Check sheet for the drawn part. Datum: minimum x, y, z corner. Units: mm. A direction names the side the tool comes from. Coordinates: 2 decimals unless noted, no trailing zeros. Order: outer loops, then holes, each group sorted by start corner. A loop starts at its lowest first (then second) coordinate and runs counter-clockwise, first axis right, second up. Notation, with made-up numbers: M 45.5,-7 L 96.5,-7 A18 ccw 96.5,25 Z; hole C 68,-12.5 d3. An arc over 180 degrees is marked long. Return JSON: item names as keys, results as strings. Group by question number.
Q1. Section check C-C, the plane x = 17. Enter the section's corners in (y, z).
Q2. Section check D-D, the plane y = 1. Enter the section's corners in (x, z), then the cut area to 3 significant figures.
Q3. Access from +Z, -Z, +X, -X, +Y, -Y to the whole of each face (thin tool, end or side, straight path). Record for the marked faces 1 and 2.
Q4. Go/stop test with flat-tipped pins: pin 1 Ø6 at (x, y) = (17.5, 7.5) entering from -Z; pin 2 Ø2 at (x, y) = (17, 5) entering from +Z; pin 3 Ø6 at (x, z) = (15.5, 6.5) entering from +Y. Record where each tip stops, or that it passes through.
Q5. Thickness scan on probe 1 along X at (y, z) = (13, 14.7); probe 2 along Y at (x, z) = (7, 14.6); probe 3 along X at (y, z) = (1.15, 7). Record the ranges inside material, lowest first.
Q6. Section check A-A, the plane y = 13. Enter the section's corners in (x, z).
Q7. Section check B-B, the plane z = 7. Enter the section's corners in (x, y).
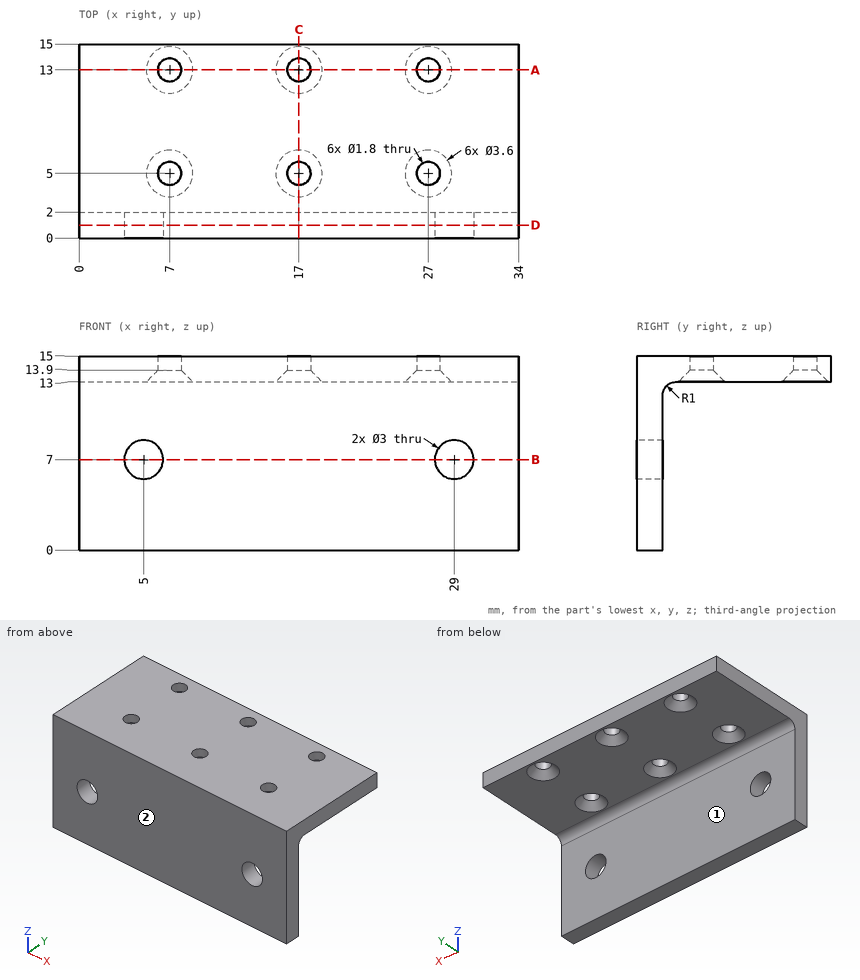
Numbers:
{
 "1": {"outline": "M 0,0 L 2,0 L 2,12 A1 cw 3,13 L 3.2,13 L 4.1,13.9 L 4.1,15 L 0,15 Z; M 5.9,13.9 L 6.8,13 L 11.2,13 L 12.1,13.9 L 12.1,15 L 5.9,15 Z; M 13.9,13.9 L 14.8,13 L 15,13 L 15,15 L 13.9,15 Z"},
 "2": {"outline": "M 0,0 L 34,0 L 34,15 L 0,15 Z; hole C 5,7 d3; hole C 29,7 d3", "area": "496 mm2"},
 "3": {"face 1": "-Z, +X, -X, +Y", "face 2": "+Z, -Z, +X, -X, -Y"},
 "4": {"pin 1": "stops at z = 13", "pin 2": "stops at z = 15", "pin 3": "stops at y = 2"},
 "5": {"probe 1": "x = 0 to 6.1, 7.9 to 16.1, 17.9 to 26.1, 27.9 to 34", "probe 2": "y = 0 to 4.1, 5.9 to 12.1, 13.9 to 15", "probe 3": "x = 0 to 3.5, 6.5 to 27.5, 30.5 to 34"},
 "6": {"outline": "M 0,13 L 5.2,13 L 6.1,13.9 L 6.1,15 L 0,15 Z; M 7.9,13.9 L 8.8,13 L 15.2,13 L 16.1,13.9 L 16.1,15 L 7.9,15 Z; M 17.9,13.9 L 18.8,13 L 25.2,13 L 26.1,13.9 L 26.1,15 L 17.9,15 Z; M 27.9,13.9 L 28.8,13 L 34,13 L 34,15 L 27.9,15 Z"},
 "7": {"outline": "M 0,0 L 3.5,0 L 3.5,2 L 0,2 Z; M 6.5,0 L 27.5,0 L 27.5,2 L 6.5,2 Z; M 30.5,0 L 34,0 L 34,2 L 30.5,2 Z"}
}
